```python
from build123d import *

# Parameters (mm, degrees)
SKETCH_3_R         = 8
SKETCH_3_R_2       = 4
EXTRUDE_716_DEPTH  = 12
EXTRUDE_1137_DEPTH = 6
SKETCH_7_W         = 140
SKETCH_7_H         = 30
EXTRUDE_1364_DEPTH = 4


with BuildPart() as part:
    # 草图3 → Extrude 716 (new body)
    with BuildSketch(Plane.XY):
        Circle(SKETCH_3_R)
        Circle(SKETCH_3_R_2, mode=Mode.SUBTRACT)
    extrude(amount=EXTRUDE_716_DEPTH)

    # 草图6 → Extrude 1137 (add)
    with BuildSketch(Plane.XY):
        with BuildLine():
            Line((-40.169068564, -125), (-33.957411481, -125))
            Line((-33.957411481, -125), (-2.5, -7.599342077))
            ThreePointArc((-2.5, -7.599342077), (-5.502602373, -5.807010171), (-7.45385736, -2.905169608))
            Line((-7.45385736, -2.905169608), (-40.169068564, -125))
        make_face()
    extrude_1137 = extrude(amount=EXTRUDE_1137_DEPTH)

    # Mirror 1200: Extrude 1137 across plane
    add(extrude_1137.mirror(Plane(origin=(0, 0, 0), x_dir=(0, 0, 1), z_dir=(1, 0, 0))))

    # 草图7 → Extrude 1364 (add)
    with BuildSketch(Plane.XZ.offset(125)):
        with Locations((0, 15)):
            Rectangle(SKETCH_7_W, SKETCH_7_H)
    extrude(amount=EXTRUDE_1364_DEPTH)


solid = part.part
```
Build history of the part. All positions in model axes, mm. A direction names the side the tool comes from. Give positions to 0.01 mm unless a question says otherwise; leave off trailing zeros. Loops run counter-clockwise (first coordinate to the right, second up) from the corner with the lowest first, then second, coordinate; pieces in that order, holes last.
Item 1: Slice it at C-C, the plane z = 3.5. List the corners of the cut face in (x, y).
Answers follow:
outline: (-70, -129) - (70, -129) - (70, -125) - (40.17, -125) - (7.45, -2.91) arc R8 ccw (long way) to (-7.45, -2.91) - (-40.17, -125) - (-70, -125) - close; hole (-33.96, -125) - (33.96, -125) - (2.5, -7.6) arc R8 cw to (-2.5, -7.6) - close; hole circle Ø8 at (0, 0)
Item 2: Slice it at A-A, the plane x = 0. List the corners of the cut face in (y, z).
Answers follow:
outline: (-129, 0) - (-125, 0) - (-125, 30) - (-129, 30) - close; (-8, 0) - (-4, 0) - (-4, 12) - (-8, 12) - close; (4, 0) - (8, 0) - (8, 12) - (4, 12) - close
Item 3: Drill centre lines: line 1 (Y direction, x = 0, z = 6.25); line 2 (Z direction, x = -23, y = -77); line 3 (Y direction, x = 37, z = 7.5). Where is each one in solid material? Low to high.
Answers follow:
line 1: y = -129 to -125, -8 to -4, 4 to 8
line 2: z = 0 to 6
line 3: y = -129 to -125
Item 4: Slice it at B-B, the plane y = 0. List the corners of the cut face in (x, z).
Answers follow:
outline: (-8, 0) - (-4, 0) - (-4, 12) - (-8, 12) - close; (4, 0) - (8, 0) - (8, 12) - (4, 12) - close
Item 5: Which spindle directions (+Z, -Z, +X, -X, +Y, -Y) get a long thin tool onto all of the face, cutting with end or side? Do faces 5 (the face through (-1, -129, 15)), 6 (the face through (-4, -2, 12)), 7 (the face through (-18.45, -67.12, 2.96)). Say none if no direction does.
Answers follow:
face 5: +Z, -Z, +X, -X, -Y
face 6: +Z, +X, -X, +Y
face 7: +Z, -Z
Item 6: Flat gauge pins, fed straight in: pin 1 (5 mm diameter, centred on y = -45, z = 7.5, fed in from +X); pin 2 (19 mm diameter, centred on x = 20, y = -69.5, fed in from +Z); pin 3 (8 mm diameter, centred on x = 2, y = -0.5, fed in from +Z); pin 4 (7 mm diameter, centred on x = 0, y = 0, fed in from +Z). Where does each tip first touch, or does it go through?
Answers follow:
pin 1: stops at x = 19.27
pin 2: stops at z = 6
pin 3: stops at z = 12
pin 4: passes through
Item 7: Slice it at D-D, the plane x = -32. List the corners of the cut face in (y, z).
Answers follow:
outline: (-129, 0) - (-125, 0) - (-125, 30) - (-129, 30) - close; (-117.69, 0) - (-94.51, 0) - (-94.51, 6) - (-117.69, 6) - close
Item 8: Pull direction X, two halves, no side cores. Call faces 1 (the face through (18.45, -67.12, 2.96)), 2 (the face through (-1, -127, 30)), 3 (the face through (-0.867, -3.905, 5.916)), 4 (the face through (23.582, -63.098, 2.958)): released by +X, released by -X, zero draft, split by the parting line, or undercut.
Answers follow:
face 1: undercut
face 2: zero draft
face 3: undercut
face 4: released by +X
